Could you check a few things on this model? Use its own coordinates, in mm. A direction names the side the tool comes from. Round coordinates to 2 decimals unless told otherwise and drop trailing zeros. Loops run counter-clockwise (first coordinate to the right, second up) from the corner with the lowest first, then second, coordinate; pieces in that order, holes last. Notation, with made-up numbers: (-6.5, 69.5) -> (18.5, 69.5) arc R15 ccw to (18.5, 80.5) -> close; hole circle Ø1 at (-0.75, -6). An arc over 180 degrees is marked (long way). One line per item, written item: value.
```python
from build123d import *

# Parameters (mm, degrees)
RESSALTO_EXTRUS_O1_DEPTH         = 7
ESBO_O2_R                        = 7.5
RESSALTO_EXTRUS_O2_DEPTH         = 1
FURO_ROSCADO_DE_M121_D           = 10.2
FURO_ROSCADO_DE_M121_CSINK_D     = 12.05
FURO_ROSCADO_DE_M121_CSINK_ANGLE = 90
FILETE1_R                        = 1
FILETE2_R                        = 1.5
CHANFRO1_SIZE                    = 0.5


# Read off the part's stored shape, not the designer's step: Furo roscado de M32
with BuildPart() as part:
    # Esboço1 → Ressalto-extrusão1 (new body)
    with BuildSketch(Plane(origin=(0, 0, 0), x_dir=(1, 0, 0), z_dir=(0, 1, 0))):
        with BuildLine():
            Line((5.123475383, 8), (-5.123475383, 8))
            ThreePointArc((-5.123475383, 8), (-6.717514421, 6.717514421), (-8, 5.123475383))
            Line((-8, 5.123475383), (-8, -5.123475383))
            ThreePointArc((-8, -5.123475383), (-6.717514421, -6.717514421), (-5.123475383, -8))
            Line((-5.123475383, -8), (5.123475383, -8))
            ThreePointArc((5.123475383, -8), (6.717514421, -6.717514421), (8, -5.123475383))
            Line((8, -5.123475383), (8, 5.123475383))
            ThreePointArc((8, 5.123475383), (6.717514421, 6.717514421), (5.123475383, 8))
        make_face()
    extrude(amount=RESSALTO_EXTRUS_O1_DEPTH)

    # Esboço2 → Ressalto-extrusão2 (add)
    with BuildSketch(Plane(origin=(0, 7, 0), x_dir=(1, 0, 0), z_dir=(0, 1, 0))):
        with Locations(Location((0, 0, 0), (0, 0, 270))):
            Circle(ESBO_O2_R)
    extrude(amount=RESSALTO_EXTRUS_O2_DEPTH)

    # Furo roscado de M121 (through all)
    with Locations(Plane(origin=(0, 8, 0), x_dir=(1, 0, 0), z_dir=(0, 1, 0))):
        with Locations((0, 0)):
            CounterSinkHole(FURO_ROSCADO_DE_M121_D / 2, FURO_ROSCADO_DE_M121_CSINK_D / 2, counter_sink_angle=FURO_ROSCADO_DE_M121_CSINK_ANGLE)

    # Filete1
    filete1_edges = [part.edges().sort_by_distance(p)[0] for p in [
        (6.717514421, 7, 6.717514421),
        (6.717514421, 7, -6.717514421),
        (-6.717514421, 7, -6.717514421),
        (-6.717514421, 7, 6.717514421),
    ]]
    fillet(filete1_edges, radius=FILETE1_R)

    # Filete2
    filete2_edges = [part.edges().sort_by_distance(p)[0] for p in [
        (6.717514421, 0, -6.717514421),
        (-6.717514421, 0, -6.717514421),
        (-6.717514421, 0, 6.717514421),
        (6.717514421, 0, 6.717514421),
    ]]
    fillet(filete2_edges, radius=FILETE2_R - 0.0001)  # a hair under: the kernel refuses the full size

    # Chanfro1
    chanfro1_edges = [part.edges().sort_by_distance(p)[0] for p in [
        (0, 8, -7.5),
    ]]
    chamfer(chanfro1_edges, length=CHANFRO1_SIZE)

    # Furo roscado de M32 outline → Furo roscado de M32 (revolve, cut)
    with BuildSketch(Plane(origin=(0, 3.5, 0), x_dir=(0.707106781186546, 0, -0.707106781186549), z_dir=(0, -1, 0))):
        Polygon((1.600067365, 9.500067365), (0, 9.500067365), (0, 4.944353867), (1.25, 4.944353867), (1.25, 9.15), align=None)
    revolve(axis=Axis((0, 3.5, 0), (0.707106781186549, 0, 0.707106781186546)), mode=Mode.SUBTRACT)


solid = part.part
```
(1) Please list where these lines run through material, in increasing order: L1, parallel to Y at x = 2.75, z = 7.5; L2, parallel to X at y = 6.25, z = 4.5; L3, parallel to Z at x = -2.5, y = 3.75.
Results below:
L1: y = 0 to 7
L2: x = -8 to -2.4, 2.4 to 8
L3: z = -8 to -4.45, 4.45 to 8
(2) We'd pull the mould along X, two halves only. Please class faces 1 (the face through (0.33, 7.246, -7.493)), 2 (the face through (-8, 3, 0)), 3 (the face through (5.41, 2.391, 4.595)): +X half, -X half, draft (parallel to the pull), parting line (faces both ways), or undercut.
Results below:
face 1: parting line
face 2: -X half
face 3: undercut
(3) Imagine slicing it at B-B on y = 0.75. Write out the boundary of the cut face in (x, z), then the cut area to 3 significant figures.
Results below:
outline: (-8, -4.74) arc R9.3 ccw to (-4.74, -8) -> (4.74, -8) arc R9.3 ccw to (8, -4.74) -> (8, 4.74) arc R9.3 ccw to (4.74, 8) -> (-4.74, 8) arc R9.3 ccw to (-8, 4.74) -> close; hole circle Ø10.2 at (0, 0)
area: 157 mm²
(4) On a 3-axis mill with a long thin cutter (end or side, diameter ignored), from which of +Z, -Z, +X, -X, +Y, -Y can I reach the whole of each face in a straight line? I mean faces 4 (the face through (5, 7, -6)), 5 (the face through (-4.864, 3.488, -1.532)). Say none if no direction works.
Results below:
face 4: +Y
face 5: +Y, -Y
(5) For pin 1 Ø3 at (x, z) = (-4, -4) entering from -Y; pin 2 Ø8 at (x, z) = (0, 0) entering from -Y, each with a flat end and sliding along its axis, tell me the tip position at first contact or that it passes through.
Results below:
pin 1: stops at y = 0
pin 2: passes through
(6) Imagine slicing it at A-A on y = 5.75. Write out the boundary of the cut face in (x, z), then the cut area to 3 significant figures.
Results below:
outline: (-8, -5.12) arc R9.5 ccw to (-5.12, -8) -> (5.12, -8) arc R9.5 ccw to (8, -5.12) -> (8, 5.12) arc R9.5 ccw to (5.12, 8) -> (-5.12, 8) arc R9.5 ccw to (-8, 5.12) -> close; hole circle Ø10.2 at (0, 0)
area: 160 mm²
